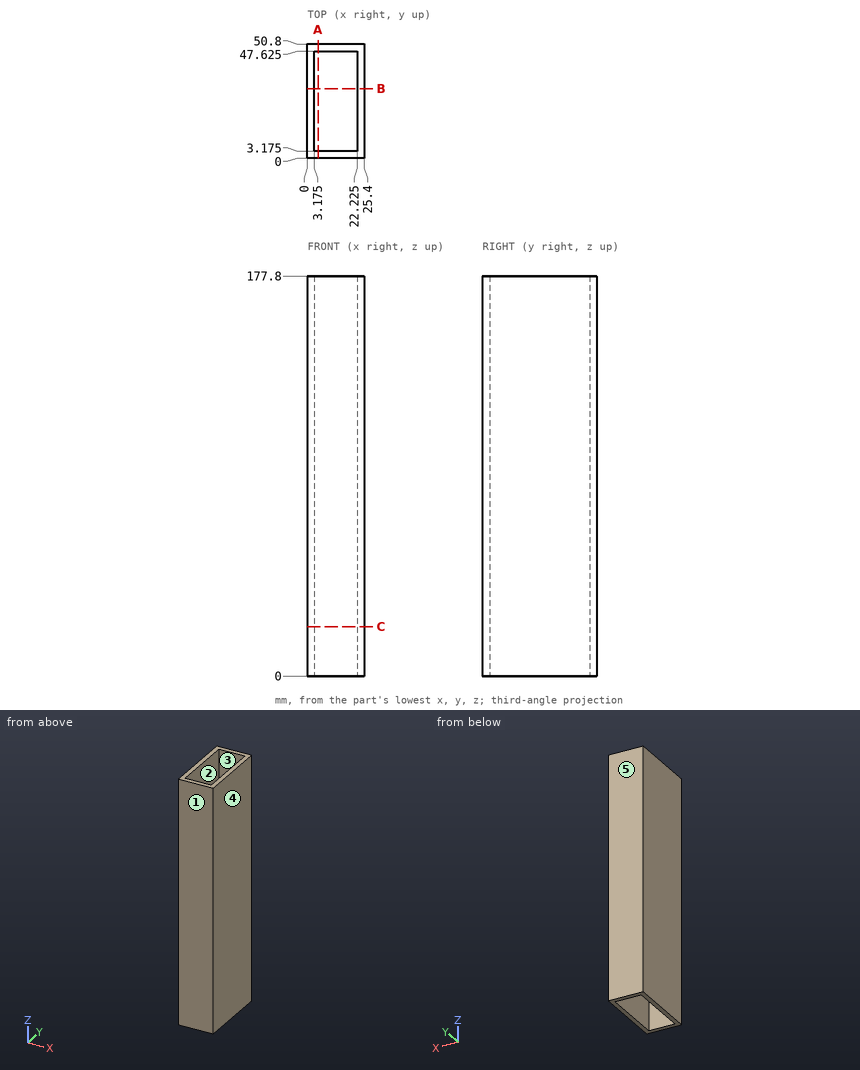
The drawing under review shows one solid part. Ordinate dimensions are in mm from its lowest x, y, z. A direction names the side the tool comes from. Coordinates: 2 decimals unless noted, no trailing zeros. Order: outer loops, then holes, each group sorted by start corner. A loop starts at its lowest first (then second) coordinate and runs counter-clockwise, first axis right, second up. Notation, with made-up numbers: (50, 64) -> (72, 64) arc R28 ccw to (72, 103) -> close; hole circle Ø4 at (-16, 19). An arc over 180 degrees is marked (long way). Return JSON: item names as keys, results as strings.
1. We need section C-C on z = 22. Write out the cut boundary in (x, y) (3 decimals), and give its area (3 significant figures).
Answer block:
{"outline": "(0, 0) -> (25.4, 0) -> (25.4, 50.8) -> (0, 50.8) -> close; hole (3.175, 3.175) -> (22.225, 3.175) -> (22.225, 47.625) -> (3.175, 47.625) -> close", "area": "444 mm²"}
2. The part is to be moulded in two halves that separate along X. For the marked faces 3, 4 and 5, say which applies: +X half, -X half, draft (parallel to the pull), parting line (faces both ways), or undercut.
Answer block:
{"face 3": "undercut", "face 4": "+X half", "face 5": "draft"}
3. Machinability: for the marked faces 1 and 2, which of the approach directions +Z, -Z, +X, -X, +Y, -Y give a long, thin tool a straight path to every point of the face, cutting with its end or side? Answer none if there is none.
Answer block:
{"face 1": "+Z, -Z, +X, -X, -Y", "face 2": "+Z, -Z"}
4. For line 1 (Y direction, x = 3.5, z = 9.5) (3 decimals); line 2 (X direction, y = 16, z = 62.5) (3 decimals), list the stretches that pass through material, from the lowest coordinate up. Write a range as from..to.
Answer block:
{"line 1": "0..3.175, 47.625..50.8", "line 2": "0..3.175, 22.225..25.4"}
5. We need section A-A on x = 4.75. Write out the cut boundary in (y, z) (3 decimals).
Answer block:
{"outline": "(0, 0) -> (3.175, 0) -> (3.175, 177.8) -> (0, 177.8) -> close; (47.625, 0) -> (50.8, 0) -> (50.8, 177.8) -> (47.625, 177.8) -> close"}
6. We need section B-B on y = 31. Write out the cut boundary in (x, z) (3 decimals), and give its area (3 significant figures).
Answer block:
{"outline": "(0, 0) -> (3.175, 0) -> (3.175, 177.8) -> (0, 177.8) -> close; (22.225, 0) -> (25.4, 0) -> (25.4, 177.8) -> (22.225, 177.8) -> close", "area": "1,130 mm²"}
